```python
from build123d import *

# Parameters (mm, degrees)
F0_R     = 25.296615
F1_DEPTH = 84.328
F2_T     = -2.54
F3_W     = 6.888267
F3_H     = 19.285627
F4_DEPTH = 25.4


with BuildPart() as f1:
    # F0 (on Front) → F1 (new body)
    with BuildSketch(Plane.XZ):
        Circle(F0_R)
    extrude(amount=F1_DEPTH)

    # F2
    f2_openings = [f1.faces().sort_by_distance(p)[0] for p in [
        (0, -84.328, 0),
    ]]
    offset(amount=F2_T, openings=f2_openings)

    # F3 (on Top) → F4 (cut)
    with BuildSketch(Plane.XY):
        with Locations((3.444133, -11.754679)):
            Rectangle(F3_W, F3_H)
    extrude(amount=-F4_DEPTH, mode=Mode.SUBTRACT)


solid = f1.part
```
CAD build for the part. Positions are in the model's coordinates, mm. A direction names the side the tool comes from. Coordinates: 2 decimals unless noted, no trailing zeros. Order: outer loops, then holes, each group sorted by start corner. A loop starts at its lowest first (then second) coordinate and runs counter-clockwise, first axis right, second up. Notation, with made-up numbers: (45, 84.25) -> (95, 84.25) arc R31 ccw to (95, 122.25) -> close; hole circle Ø8 at (56, 33.25). An arc over 180 degrees is marked (long way). Use one line per item in the form item = value. Start each with the question number.
1) Band-saw the part on B-B on y = -27. Give the cut face in (x, z).
2) Band-saw the part on A-A on x = 2.5. Give the cut face in (y, z), then the cut area to 3 significant figures.
3) Tool access for faces 4 (the flat face through (-0.3, -2.54, 0.3)), 5 (the flat face through (0, -10, -23)), 6 (the flat face through (-23, -84.328, 4)): list every direction of +Z, -Z, +X, -X, +Y, -Y with a clear straight run to the whole face (end or side of a thin tool).
4) Drill centre lines: L1, parallel to Z at x = 0, y = -65; L2, parallel to Y at x = 10, z = 10; L3, parallel to Z at x = -19, y = -8.5. Where is each one in solid material? Low to high. Write a range as [from, to].
5) Pull direction X, two halves, no side cores. Call faces 1 (the flat face through (0, 0, 0)), 2 (the flat face through (3, -21.397, -24)), 3 (the cylindrical face through (23.368, -41.574, -9.689)): +X half, -X half, draft (parallel to the pull), parting line (faces both ways), or undercut.
6) Drop flat-ended pins along their axis: pin 1 (9.5 mm diameter, centred on y = -12, z = -13, fed in from +X); pin 2 (3.5 mm diameter, centred on x = 5, z = -19, fed in from -Y); pin 3 (2 mm diameter, centred on y = -68, z = -8.5, fed in from -X); pin 4 (8 mm diameter, centred on x = -9.5, z = -12, fed in from +Y). Give the stop position or say it passes through.
7) Band-saw the part on D-D on x = -14. Give the cut face in (y, z), then the cut area to 3 significant figures.
8) Band-saw the part on C-C on z = 8. Give the cut face in (x, y), then the cut area to 3 significant figures.
Entries:
q1.outline = circle Ø50.59 at (0, 0); hole circle Ø45.51 at (0, 0)
q2.outline = (-84.33, -25.17) -> (-21.4, -25.17) -> (-21.4, -22.62) -> (-84.33, -22.62) -> close; (-84.33, 22.62) -> (-2.54, 22.62) -> (-2.54, 0) -> (-2.11, 0) -> (-2.11, -25.17) -> (0, -25.17) -> (0, 25.17) -> (-84.33, 25.17) -> close
q2.area = 487 mm2
q3.face_4 = -Y
q3.face_5 = -Z
q3.face_6 = +Z, -Z, +X, -X, -Y
q4.L1 = [-25.3, -22.76], [22.76, 25.3]
q4.L2 = [-2.54, 0]
q4.L3 = [-16.7, -12.52], [12.52, 16.7]
q5.face_1 = draft
q5.face_2 = undercut
q5.face_3 = parting line
q6.pin_1 = 23.91
q6.pin_2 = -2.11
q6.pin_3 = -24.16
q6.pin_4 = 0
q7.outline = (-84.33, -21.07) -> (0, -21.07) -> (0, 21.07) -> (-84.33, 21.07) -> (-84.33, 17.94) -> (-2.54, 17.94) -> (-2.54, -17.94) -> (-84.33, -17.94) -> close
q7.area = 619 mm2
q8.outline = (-24, -84.33) -> (-21.3, -84.33) -> (-21.3, -2.54) -> (21.3, -2.54) -> (21.3, -84.33) -> (24, -84.33) -> (24, 0) -> (-24, 0) -> close
q8.area = 563 mm2
